Part model, mm, in its own coordinate system. Face numbers are marked on the shaded views. Coordinates: 2 decimals unless noted, no trailing zeros. Loops run counter-clockwise (first coordinate to the right, second up) from the corner with the lowest first, then second, coordinate; pieces in that order, holes last. Notation, with made-up numbers: (61, 1) -> (100, 1) arc R10 cw to (100, 8) -> close; hole circle Ø11 at (-20, 10). An arc over 180 degrees is marked (long way). Use one line per item in the form item = value. Start each with the question number.
(1) Band-saw the part on C-C on z = 6.75. Give the cut face in (x, y).
(2) Band-saw the part on B-B on x = 63. Give the cut face in (y, z).
(3) Pin check, flat tip, straight feed: P1, Ø3, axis at x = 77.5, y = 9, coming from the +Z side. Stop position of the tip, or through.
(4) Band-saw the part on A-A on y = 22. Give the cut face in (x, z), then the cut area to 3 significant figures.
(5) Mould opens along Y. For the marked faces 1 and 2 say: +Y half, -Y half, draft (parallel to the pull), parting line (faces both ways), or undercut.
(6) Drill centre lines: L1, parallel to Y at x = -12.5, z = 6.5; L2, parallel to X at y = 11, z = 5; L3, parallel to Z at x = -18, y = 56.5. Where is each one in solid material? Low to high. Write a range as [from, to].
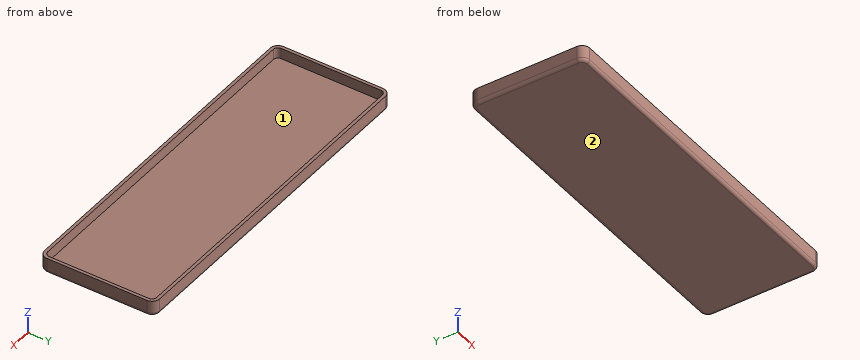
```python
from build123d import *

# Parameters (mm, degrees)
F1_DEPTH = 3
F2_DEPTH = 10
F3_R     = 2


# Not quite as in the source:
# - a feature names something its author has since deleted; it is built from what else it names


with BuildPart() as f1:
    # F0 (on Top) → F1 (new body)
    with BuildSketch(Plane.XY):
        with BuildLine():
            ThreePointArc((-44.6118305922, 5), (-43.7331509357, 2.8786796564), (-41.6118305922, 2))
            Line((-41.6118305922, 2), (173.3881694078, 2))
            ThreePointArc((173.3881694078, 2), (175.5094897514, 2.8786796564), (176.3881694078, 5))
            Line((176.3881694078, 5), (176.3881694078, 70))
            ThreePointArc((176.3881694078, 70), (175.5094897514, 72.1213203436), (173.3881694078, 73))
            Line((173.3881694078, 73), (-41.6118305922, 73))
            ThreePointArc((-41.6118305922, 73), (-43.7331509357, 72.1213203436), (-44.6118305922, 70))
            Line((-44.6118305922, 70), (-44.6118305922, 5))
        make_face()
    extrude(amount=F1_DEPTH)

    # F0 (on Top) → F2 (join)
    with BuildSketch(Plane.XY):
        with BuildLine():
            Line((173.3881694078, 75), (-41.6118305922, 75))
            ThreePointArc((-41.6118305922, 75), (-45.1473644981, 73.5355339059), (-46.6118305922, 70))
            Line((-46.6118305922, 70), (-46.6118305922, 5))
            ThreePointArc((-46.6118305922, 5), (-45.1473644981, 1.4644660941), (-41.6118305922, 0))
            Line((-41.6118305922, 0), (173.3881694078, 0))
            ThreePointArc((173.3881694078, 0), (176.9237033138, 1.4644660941), (178.3881694078, 5))
            Line((178.3881694078, 5), (178.3881694078, 70))
            ThreePointArc((178.3881694078, 70), (176.9237033138, 73.5355339059), (173.3881694078, 75))
        make_face()
        with BuildLine():
            Line((173.3881694078, 2), (-41.6118305922, 2))
            ThreePointArc((-41.6118305922, 2), (-43.7331509357, 2.8786796564), (-44.6118305922, 5))
            Line((-44.6118305922, 5), (-44.6118305922, 70))
            ThreePointArc((-44.6118305922, 70), (-43.7331509357, 72.1213203436), (-41.6118305922, 73))
            Line((-41.6118305922, 73), (173.3881694078, 73))
            ThreePointArc((173.3881694078, 73), (175.5094897514, 72.1213203436), (176.3881694078, 70))
            Line((176.3881694078, 70), (176.3881694078, 5))
            ThreePointArc((176.3881694078, 5), (175.5094897514, 2.8786796564), (173.3881694078, 2))
        make_face(mode=Mode.SUBTRACT)
    extrude(amount=F2_DEPTH)

    # F3
    f3_edges = [f1.edges().sort_by_distance(p)[0] for p in [
        (65.888169, 75, 0),
    ]]
    fillet(f3_edges, radius=F3_R)


solid = f1.part
```
A:
q1.outline = (-46.61, 5) arc R5 ccw to (-41.61, 0) -> (173.39, 0) arc R5 ccw to (178.39, 5) -> (178.39, 70) arc R5 ccw to (173.39, 75) -> (-41.61, 75) arc R5 ccw to (-46.61, 70) -> close; hole (-44.61, 5) arc R3 ccw to (-41.61, 2) -> (173.39, 2) arc R3 ccw to (176.39, 5) -> (176.39, 70) arc R3 ccw to (173.39, 73) -> (-41.61, 73) arc R3 ccw to (-44.61, 70) -> close
q2.outline = (0, 2) arc R2 ccw to (2, 0) -> (73, 0) arc R2 ccw to (75, 2) -> (75, 10) -> (73, 10) -> (73, 3) -> (2, 3) -> (2, 10) -> (0, 10) -> close
q3.P1 = 3
q4.outline = (-46.61, 2) arc R2 ccw to (-44.61, 0) -> (176.39, 0) arc R2 ccw to (178.39, 2) -> (178.39, 10) -> (176.39, 10) -> (176.39, 3) -> (-44.61, 3) -> (-44.61, 10) -> (-46.61, 10) -> close
q4.area = 701 mm²
q5.face_1 = undercut
q5.face_2 = draft
q6.L1 = [0, 2], [73, 75]
q6.L2 = [-46.61, -44.61], [176.39, 178.39]
q6.L3 = [0, 3]
